Autodesk Inventor part; units mm, degrees
ref_plane "YZ Plane" through (0, 0, 0) normal (1, 0, 0) x (0, 1, 0)
ref_plane "XZ Plane" through (0, 0, 0) normal (0, 1, 0) x (-1, 0, 0)
ref_plane "XY Plane" through (0, 0, 0) normal (0, 0, 1) x (1, 0, 0)
sketch "Sketch2" plane through (0, 0, 0) normal (0, 0, 1) x (1, 0, 0)
  line L0 (0, 0) -> (31.75, 0)
  line L1 (31.75, 0) -> (31.75, 31.75)
  line L2 (31.75, 31.75) -> (0, 31.75)
  line L3 (0, 31.75) -> (0, 0)
  line L4 (2, 29.75) -> (29.75, 29.75)
  line L5 (29.75, 29.75) -> (29.75, 2)
  line L6 (29.75, 2) -> (2, 2)
  line L7 (2, 2) -> (2, 29.75)
  dimension "d0" = 31.75
  dimension "d1" = 31.75
  dimension "d2" = 2
extrude "Extrusion1" add sketch "Sketch2" along normal blind 1650
sketch "Sketch3" plane through (0, 0, 1650) normal (0, 0, 1) x (1, 0, 0)
  line L0 (31.75, 31.75) -> (0, 31.75)
  line L1 (0, 31.75) -> (-55.875, 31.75)
  line L2 (-55.875, 31.75) -> (-55.875, 0)
  line L3 (-55.875, 0) -> (0, 0)
  line L4 (0, 0) -> (0, 31.75)
  line L5 (31.75, 31.75) -> (87.625, 31.75)
  line L6 (87.625, 31.75) -> (87.625, 0)
  line L7 (87.625, 0) -> (31.75, 0)
  line L8 (31.75, 0) -> (31.75, 31.75)
  circle A0 centre (-40, 15.875) radius 6
  circle A1 centre (71.75, 15.875) radius 6
  dimension "d5" = 55.875
  dimension "d6" = 55.875
  dimension "d7" = 12
  dimension "d8" = 12
  dimension "d15" = 111.75
  dimension "d16" = 40
extrude "Extrusion2" add sketch "Sketch3" against normal blind 6
sketch "Sketch4" plane through (0, 0, 0) normal (0, 0, -1) x (-1, 0, 0)
  line L0 (-87.625, 31.75) -> (55.875, 31.75)
  line L1 (55.875, 0) -> (-87.625, 0)
  line L2 (40, 31.75) -> (55.875, 31.75)
  line L3 (55.875, 31.75) -> (55.875, 0)
  line L4 (55.875, 0) -> (25.875, 0)
  line L5 (-31.75, 31.75) -> (-31.75, 0)
  line L6 (-31.75, 31.75) -> (-87.625, 31.75)
  line L7 (-87.625, 31.75) -> (-87.625, 0)
  line L8 (-87.625, 0) -> (-31.75, 0)
  line L9 (-31.75, 0) -> (-31.75, 31.75)
  circle A0 centre (-71.75, 15.875) radius 6
  circle A1 centre (-71.75, 15.875) radius 6
  circle A2 centre (40, 15.875) radius 6
  line L10 (0, 31.75) -> (0, 0)
  point P0 (55.875, 31.75)
  point P1 (-87.625, 31.75)
  point P2 (-87.625, 0)
  point P3 (-87.625, 0)
  dimension "d11" = 55.875
  dimension "d12" = 12
  dimension "d17" = 40
  dimension "d18" = 111.75
extrude "Extrusion3" add sketch "Sketch4" against normal blind 6 contours L0 L5 L1 L7 | L0 L3 L1 L10
properties part number "Bases_MDF_Acero"
Verification items for the finished model (mm, model axes). A direction names the side the tool comes from. Give positions to 0.01 mm unless a question says otherwise; leave off trailing zeros. Write each loop counter-clockwise with the first axis right and the second up, starting at its lowest first coordinate (ties: lowest second). Pieces come first, ordered by that corner, then holes. Notation, with made-up numbers: (-0.5, 29) -> (29.5, 29) arc R17 ccw to (29.5, 53) -> close; hole circle Ø5 at (18, 59). An arc over 180 degrees is marked (long way). Use CSV: the item, a comma, the result in double quotes.
(1) Set-up check for faces 4 (the flat face through (2, 16, 813)), 5 (the flat face through (31.75, 16, 814)), 6 (the flat face through (15, 30, 0)), 7 (the flat face through (-28, 16, 1644)): record each of +Z, -Z, +X, -X, +Y, -Y from which the full face is reachable in a straight line by a thin tool's end or side.
Derived:
face 4,"+Z, -Z"
face 5,"+X, +Y, -Y"
face 6,"-Z, +X, -X, +Y, -Y"
face 7,"-X, +Y, -Y"
(2) Go/stop test with flat-tipped pins: pin 1 (2 mm diameter, centred on y = 6.5, z = 829.5, fed in from +X); pin 2 (8.5 mm diameter, centred on y = 18.5, z = 770.5, fed in from -X); pin 3 (9.5 mm diameter, centred on x = 71.75, y = 15.875, fed in from -Z). Record where each tip stops, or that it passes through.
Derived:
pin 1,"stops at x = 31.75"
pin 2,"stops at x = 0"
pin 3,"passes through"
(3) Release check for a two-part mould opening along Z. For faces 1 (the flat face through (15, 30, 1650)), 2 (the flat face through (0, 16, 814)), 3 (the flat face through (11, 31.75, 821)) record: +Z half, -Z half, draft (parallel to the pull), parting line (faces both ways), or undercut.
Derived:
face 1,"+Z half"
face 2,"undercut"
face 3,"draft"
(4) Material ranges on L1, parallel to X at y = 22.5, z = 915; L2, parallel to Y at x = 71.75, z = 2.4 (3 decimals); L3, parallel to Z at x = -44, y = 6.5, recorded low to high.
Derived:
L1,"x = 0 to 2, 29.75 to 31.75"
L2,"y = 0 to 9.875, 21.875 to 31.75"
L3,"z = 0 to 6, 1644 to 1650"
(5) Sectioned sample at B-B (z = 984.5). Record the cut outline in (x, y).
Derived:
outline,"(0, 0) -> (31.75, 0) -> (31.75, 31.75) -> (0, 31.75) -> close; hole (2, 2) -> (29.75, 2) -> (29.75, 29.75) -> (2, 29.75) -> close"
(6) Sectioned sample at A-A (x = 49.5). Record the cut outline in (y, z), plus the area to 3 significant figures.
Derived:
outline,"(0, 0) -> (31.75, 0) -> (31.75, 6) -> (0, 6) -> close; (0, 1644) -> (31.75, 1644) -> (31.75, 1650) -> (0, 1650) -> close"
area,"381 mm^2"
